Can you work these out from the model? Positions are in its coordinate system, mm. Give positions to 0.01 mm unless a question says otherwise; leave off trailing zeros. Loops run counter-clockwise (first coordinate to the right, second up) from the corner with the lowest first, then second, coordinate; pieces in that order, holes last. Notation, with made-up numbers: (55, 67.25) -> (101, 67.25) arc R9 cw to (101, 73.25) -> close; hole circle Ø3 at (0.25, 22). An arc over 180 degrees is marked (long way). Use CSV: the item, a comma, the result in double quotes.
from build123d import *

# Parameters (mm, degrees)
SKETCH_R        = 55
PAD_DEPTH       = 4
SKETCH003_R     = 1.3
POCKET001_DEPTH = 5
SKETCH004_R     = 1.3
POCKET_DEPTH    = 5


with BuildPart() as part:
    # Sketch → Pad (new body)
    with BuildSketch(Plane.XY):
        Circle(SKETCH_R)
    extrude(amount=PAD_DEPTH)

    # Sketch003 → Pocket001 (cut)
    with BuildSketch(Plane.XY.offset(4)):
        with Locations((-44, -20)):
            Circle(SKETCH003_R)
        with Locations((44, 20)):
            Circle(SKETCH003_R)
    extrude(amount=-POCKET001_DEPTH, mode=Mode.SUBTRACT)

    # Sketch004 (on Face3 of Pocket001) → Pocket (cut)
    with BuildSketch(Plane.XY.offset(4)):
        with Locations((3, -50)):
            Circle(SKETCH004_R)
        with Locations((-3, -50)):
            Circle(SKETCH004_R)
        with Locations((-3, 50)):
            Circle(SKETCH004_R)
        with Locations((3, 50)):
            Circle(SKETCH004_R)
    extrude(amount=-POCKET_DEPTH, mode=Mode.SUBTRACT)


solid = part.part
(1) If we section it at B-B, the plane y = 20: Write out the boundary of the cut face in (x, z), then the cut area to 3 significant figures.
Answer sheet:
outline,"(-51.23, 0) -> (42.7, 0) -> (42.7, 4) -> (-51.23, 4) -> close; (45.3, 0) -> (51.23, 0) -> (51.23, 4) -> (45.3, 4) -> close"
area,"399 mm2"
(2) If I drill on L1, parallel to Y at x = -3, z = 2.8; L2, parallel to Y at x = -44, z = 2.25; L3, parallel to X at y = 1.5, z = 2.7, over which ranges is the centre line in solid material (lowest first)? Write a range as from..to.
Answer sheet:
L1,"y = -54.92..-51.3, -48.7..48.7, 51.3..54.92"
L2,"y = -33..-21.3, -18.7..33"
L3,"x = -54.98..54.98"
(3) Will these pins go through, and if not, where does the flat tip stop? pin 1 Ø1 at (y, z) = (-23.5, 2) entering from -X; pin 2 Ø2 at (x, z) = (6, 2.5) entering from +Y; pin 3 Ø2 at (x, z) = (39.5, 1) entering from -Y.
Answer sheet:
pin 1,"stops at x = -49.96"
pin 2,"stops at y = 54.77"
pin 3,"stops at y = -39.28"
(4) If we section it at D-D, the plane y = -50: Write out the boundary of the cut face in (x, z).
Answer sheet:
outline,"(-22.91, 0) -> (-4.3, 0) -> (-4.3, 4) -> (-22.91, 4) -> close; (-1.7, 0) -> (1.7, 0) -> (1.7, 4) -> (-1.7, 4) -> close; (4.3, 0) -> (22.91, 0) -> (22.91, 4) -> (4.3, 4) -> close"
(5) We'd pull the mould along Y, two halves only. Please class faces 1 (the face through (2.83, 51.29, 2.03)), 2 (the face through (-1, 1, 0)), 3 (the face through (-11.923, -53.692, 1.972)): released by +Y, released by -Y, zero draft, split by the parting line, or undercut.
Answer sheet:
face 1,"undercut"
face 2,"zero draft"
face 3,"split by the parting line"
(6) If we section it at A-A, the plane x = 44: Write out the boundary of the cut face in (y, z), then the cut area to 3 significant figures.
Answer sheet:
outline,"(-33, 0) -> (18.7, 0) -> (18.7, 4) -> (-33, 4) -> close; (21.3, 0) -> (33, 0) -> (33, 4) -> (21.3, 4) -> close"
area,"254 mm2"
(7) If we section it at C-C, the plane z = 2.7: Write out the boundary of the cut face in (x, y).
Answer sheet:
outline,"circle Ø110 at (0, 0); hole circle Ø2.6 at (-44, -20); hole circle Ø2.6 at (-3, -50); hole circle Ø2.6 at (-3, 50); hole circle Ø2.6 at (3, -50); hole circle Ø2.6 at (3, 50); hole circle Ø2.6 at (44, 20)"
